Model file for the job. Use its own axes, mm. A direction names the side the tool comes from. Give positions to 0.01 mm unless a question says otherwise; leave off trailing zeros. Loops run counter-clockwise (first coordinate to the right, second up) from the corner with the lowest first, then second, coordinate; pieces in that order, holes last. Notation, with made-up numbers: (69, 78) - (86, 78) arc R28 cw to (86, 103) - close; hole circle Ø5 at (-2.5, 1). An arc over 180 degrees is marked (long way). Use a Markdown table: item, result.
from build123d import *

# Parameters (mm, degrees)
SKETCH1_R           = 3.5
BOSS_EXTRUDE1_DEPTH = 195


with BuildPart() as part:
    # Sketch1 → Boss-Extrude1 (new body)
    with BuildSketch(Plane.XY):
        with BuildLine():
            Line((-7.5, -4.671572875), (-7.5, 4.671572875))
            Line((-7.5, 4.671572875), (-12.646446609, 9.818019485))
            ThreePointArc((-12.646446609, 9.818019485), (-13.191341716, 9.92640586), (-13.5, 9.464466094))
            Line((-13.5, 9.464466094), (-13.5, 3.75))
            ThreePointArc((-13.5, 3.75), (-13.573223305, 3.573223305), (-13.75, 3.5))
            Line((-13.75, 3.5), (-17.25, 3.5))
            ThreePointArc((-17.25, 3.5), (-17.426776695, 3.573223305), (-17.5, 3.75))
            Line((-17.5, 3.75), (-17.5, 18.323223305))
            ThreePointArc((-17.5, 18.323223305), (-17.448223305, 18.448223305), (-17.323223305, 18.5))
            Line((-17.323223305, 18.5), (-3.75, 18.5))
            ThreePointArc((-3.75, 18.5), (-3.573223305, 18.426776695), (-3.5, 18.25))
            Line((-3.5, 18.25), (-3.5, 14.75))
            ThreePointArc((-3.5, 14.75), (-3.573223305, 14.573223305), (-3.75, 14.5))
            Line((-3.75, 14.5), (-10.464466094, 14.5))
            ThreePointArc((-10.464466094, 14.5), (-10.92640586, 14.191341716), (-10.818019485, 13.646446609))
            Line((-10.818019485, 13.646446609), (-4.671572875, 7.5))
            Line((-4.671572875, 7.5), (4.671572875, 7.5))
            Line((4.671572875, 7.5), (10.818019485, 13.646446609))
            ThreePointArc((10.818019485, 13.646446609), (10.92640586, 14.191341716), (10.464466094, 14.5))
            Line((10.464466094, 14.5), (3.75, 14.5))
            ThreePointArc((3.75, 14.5), (3.573223305, 14.573223305), (3.5, 14.75))
            Line((3.5, 14.75), (3.5, 18.25))
            ThreePointArc((3.5, 18.25), (3.573223305, 18.426776695), (3.75, 18.5))
            Line((3.75, 18.5), (17.323223305, 18.5))
            ThreePointArc((17.323223305, 18.5), (17.448223305, 18.448223305), (17.5, 18.323223305))
            Line((17.5, 18.323223305), (17.5, 3.75))
            ThreePointArc((17.5, 3.75), (17.426776695, 3.573223305), (17.25, 3.5))
            Line((17.25, 3.5), (13.75, 3.5))
            ThreePointArc((13.75, 3.5), (13.573223305, 3.573223305), (13.5, 3.75))
            Line((13.5, 3.75), (13.5, 9.464466094))
            ThreePointArc((13.5, 9.464466094), (13.191341716, 9.92640586), (12.646446609, 9.818019485))
            Line((12.646446609, 9.818019485), (7.5, 4.671572875))
            Line((7.5, 4.671572875), (7.5, -4.671572875))
            Line((7.5, -4.671572875), (12.646446609, -9.818019485))
            ThreePointArc((12.646446609, -9.818019485), (13.191341716, -9.92640586), (13.5, -9.464466094))
            Line((13.5, -9.464466094), (13.5, -3.75))
            ThreePointArc((13.5, -3.75), (13.573223305, -3.573223305), (13.75, -3.5))
            Line((13.75, -3.5), (17.25, -3.5))
            ThreePointArc((17.25, -3.5), (17.426776695, -3.573223305), (17.5, -3.75))
            Line((17.5, -3.75), (17.5, -18.323223305))
            ThreePointArc((17.5, -18.323223305), (17.448223305, -18.448223305), (17.323223305, -18.5))
            Line((17.323223305, -18.5), (3.75, -18.5))
            ThreePointArc((3.75, -18.5), (3.573223305, -18.426776695), (3.5, -18.25))
            Line((3.5, -18.25), (3.5, -14.75))
            ThreePointArc((3.5, -14.75), (3.573223305, -14.573223305), (3.75, -14.5))
            Line((3.75, -14.5), (10.464466094, -14.5))
            ThreePointArc((10.464466094, -14.5), (10.92640586, -14.191341716), (10.818019485, -13.646446609))
            Line((10.818019485, -13.646446609), (4.671572875, -7.5))
            Line((4.671572875, -7.5), (-4.671572875, -7.5))
            Line((-4.671572875, -7.5), (-10.818019485, -13.646446609))
            ThreePointArc((-10.818019485, -13.646446609), (-10.92640586, -14.191341716), (-10.464466094, -14.5))
            Line((-10.464466094, -14.5), (-3.75, -14.5))
            ThreePointArc((-3.75, -14.5), (-3.573223305, -14.573223305), (-3.5, -14.75))
            Line((-3.5, -14.75), (-3.5, -18.25))
            ThreePointArc((-3.5, -18.25), (-3.573223305, -18.426776695), (-3.75, -18.5))
            Line((-3.75, -18.5), (-17.323223305, -18.5))
            ThreePointArc((-17.323223305, -18.5), (-17.448223305, -18.448223305), (-17.5, -18.323223305))
            Line((-17.5, -18.323223305), (-17.5, -3.75))
            ThreePointArc((-17.5, -3.75), (-17.426776695, -3.573223305), (-17.25, -3.5))
            Line((-17.25, -3.5), (-13.75, -3.5))
            ThreePointArc((-13.75, -3.5), (-13.573223305, -3.573223305), (-13.5, -3.75))
            Line((-13.5, -3.75), (-13.5, -9.464466094))
            ThreePointArc((-13.5, -9.464466094), (-13.191341716, -9.92640586), (-12.646446609, -9.818019485))
            Line((-12.646446609, -9.818019485), (-7.5, -4.671572875))
        make_face()
        Circle(SKETCH1_R, mode=Mode.SUBTRACT)
    extrude(amount=BOSS_EXTRUDE1_DEPTH)


solid = part.part
(1) Mould opens along X. For faces 1 (the flat face through (-7.79, 10.62, 96.14)), 2 (the flat face through (-17.5, 11, 96)), 3 (the flat face through (16, 3.5, 96)) say: pulls with the +X half, pulls with the -X half, needs draft (parallel to the pull), parting line crosses it, or undercut.
Computed:
| item | result |
|---|---|
| face 1 | undercut |
| face 2 | pulls with the -X half |
| face 3 | needs draft |
(2) Slice it at A-A, the plane y = 0. Write the cut outline in (x, z).
Computed:
| item | result |
|---|---|
| outline | (-7.5, 0) - (-3.5, 0) - (-3.5, 195) - (-7.5, 195) - close; (3.5, 0) - (7.5, 0) - (7.5, 195) - (3.5, 195) - close |
(3) 3-axis set-ups, long thin cutter, end or side, ignore diameter. For faces 4 (the flat face through (13.5, -7, 96)), 5 (the flat face through (3.5, 16, 96)), 6 (the flat face through (3.5, -17, 96)), 7 (the flat face through (-16, -3.5, 96)), 8 (the flat face through (17.5, -11, 96)): which of +Z, -Z, +X, -X, +Y, -Y reach the whole face in a straight line?
Computed:
| item | result |
|---|---|
| face 4 | +Z, -Z |
| face 5 | +Z, -Z, +Y |
| face 6 | +Z, -Z, -Y |
| face 7 | +Z, -Z, -X |
| face 8 | +Z, -Z, +X, +Y, -Y |
(4) Pin check, flat tips, straight feed: P1, Ø4.5, axis at y = 0.5, z = 133, coming from the +X side; P2, Ø1.5, axis at x = -8.5, y = 10, coming from the -Z side. Stop position of each tip, or through.
Computed:
| item | result |
|---|---|
| P1 | x = 7.5 |
| P2 | z = 0 |
(5) Drill centre lines: probe 1 along Y at (x, z) = (-4.5, 56); probe 2 along Y at (x, z) = (0, 87); probe 3 along X at (y, z) = (-5, 106). Where is each one in solid material? Low to high. Write a range as [from, to].
Computed:
| item | result |
|---|---|
| probe 1 | [-18.5, -14.5], [-7.5, 7.5], [14.5, 18.5] |
| probe 2 | [-7.5, -3.5], [3.5, 7.5] |
| probe 3 | [-17.5, -13.5], [-7.83, 7.83], [13.5, 17.5] |
